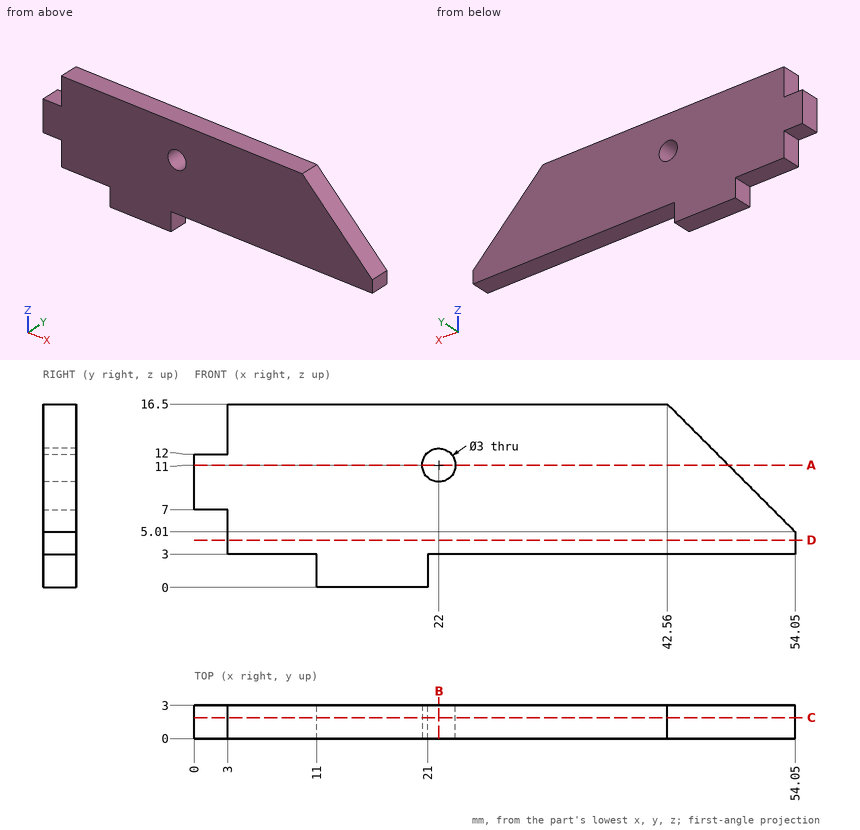
Verification items for this drawing (mm, ordinates from the low corner). Round coordinates to 2 decimals unless told otherwise and drop trailing zeros. Loops run counter-clockwise (first coordinate to the right, second up) from the corner with the lowest first, then second, coordinate; pieces in that order, holes last. Notation, with made-up numbers: (58.5, 1.5) -> (115.5, 1.5) arc R8 ccw to (115.5, 14.5) -> close; hole circle Ø5 at (25, 82). An arc over 180 degrees is marked (long way). Answer in a Markdown table with one row per item.
Q1. Go/stop test with flat-tipped pins: P1, Ø0.9, axis at y = 1.5, z = 6, coming from the -X side; P2, Ø0.9, axis at x = 2, y = 1.5, coming from the -Z side; P3, Ø2.5, axis at x = 22, z = 11, coming from the -Y side; P4, Ø0.9, axis at x = 1, y = 2, coming from the +Z side. Record where each tip stops, or that it passes through.
Data:
| item | result |
|---|---|
| P1 | stops at x = 3 |
| P2 | stops at z = 7 |
| P3 | passes through |
| P4 | stops at z = 12 |
Q2. Sectioned sample at B-B on x = 22. Enter the section's corners in (y, z).
Data:
| item | result |
|---|---|
| outline | (0, 3) -> (3, 3) -> (3, 9.5) -> (0, 9.5) -> close; (0, 12.5) -> (3, 12.5) -> (3, 16.5) -> (0, 16.5) -> close |
Q3. Sectioned sample at D-D on z = 4.25. Enter the section's corners in (x, y), then the cut area to 3 significant figures.
Data:
| item | result |
|---|---|
| outline | (3, 0) -> (54.05, 0) -> (54.05, 3) -> (3, 3) -> close |
| area | 153 mm^2 |
Q4. Sectioned sample at A-A on z = 11. Enter the section's corners in (x, y).
Data:
| item | result |
|---|---|
| outline | (0, 0) -> (20.5, 0) -> (20.5, 3) -> (0, 3) -> close; (23.5, 0) -> (48.06, 0) -> (48.06, 3) -> (23.5, 3) -> close |
Q5. Sectioned sample at C-C on y = 1.9. Enter the section's corners in (x, z), then the cut area to 3 significant figures.
Data:
| item | result |
|---|---|
| outline | (0, 7) -> (3, 7) -> (3, 3) -> (11, 3) -> (11, 0) -> (21, 0) -> (21, 3) -> (54.05, 3) -> (54.05, 5.01) -> (42.56, 16.5) -> (3, 16.5) -> (3, 12) -> (0, 12) -> close; hole circle Ø3 at (22, 11) |
| area | 661 mm^2 |
Q6. Thickness scan on L1, parallel to Z at x = 22, y = 0.7; L2, parallel to X at y = 0.65, z = 1.75; L3, parallel to Z at x = 30, y = 2.3. Record the ranges inside material, lowest first.
Data:
| item | result |
|---|---|
| L1 | z = 3 to 9.5, 12.5 to 16.5 |
| L2 | x = 11 to 21 |
| L3 | z = 3 to 16.5 |
